```python
from build123d import *

# Parameters (mm, degrees)
SKETCH_1_W      = 27.5
SKETCH_1_H      = 13.5
EXTRUDE_1_DEPTH = 2.5
SKETCH_2_W      = 2.5
SKETCH_2_H      = 13.5
EXTRUDE_2_DEPTH = 3
SKETCH_3_R      = 0.25
EXTRUDE_3_DEPTH = 3
SKETCH_4_R      = 0.25
SKETCH_4_R_2    = 2.5
EXTRUDE_5_DEPTH = 20


with BuildPart() as part:
    # Эскиз1 → Бобышка-Вытянуть1 (new body)
    with BuildSketch(Plane(origin=(0, 0, 0), x_dir=(1, 0, 0), z_dir=(0, 1, 0))):
        Rectangle(SKETCH_1_W, SKETCH_1_H)
    extrude(amount=EXTRUDE_1_DEPTH)

    # Эскиз2 → Бобышка-Вытянуть2 (add)
    with BuildSketch(Plane.XZ):
        with Locations((12.5, 0)):
            Rectangle(SKETCH_2_W, SKETCH_2_H)
    extrude(amount=-EXTRUDE_2_DEPTH)

    # Эскиз3 → Бобышка-Вытянуть3 (add)
    with BuildSketch(Plane.ZY.offset(13.75)):
        with Locations(Location((1.75, 1.25, 0), (0, 0, 180))):
            Circle(SKETCH_3_R)
    extrude(amount=EXTRUDE_3_DEPTH)

    # Эскиз4 → Бобышка-Вытянуть5 (add)
    with BuildSketch(Plane.ZY.offset(16.75)):
        with Locations(Location((1.75, 1.25, 0), (0, 0, 180))):
            Circle(SKETCH_4_R)
        with Locations((-0.5, 1.25)):
            Circle(SKETCH_4_R_2)
        with Locations(Location((1.75, 1.25, 0), (0, 0, 180))):
            Circle(SKETCH_4_R)
    extrude(amount=EXTRUDE_5_DEPTH)


solid = part.part
```
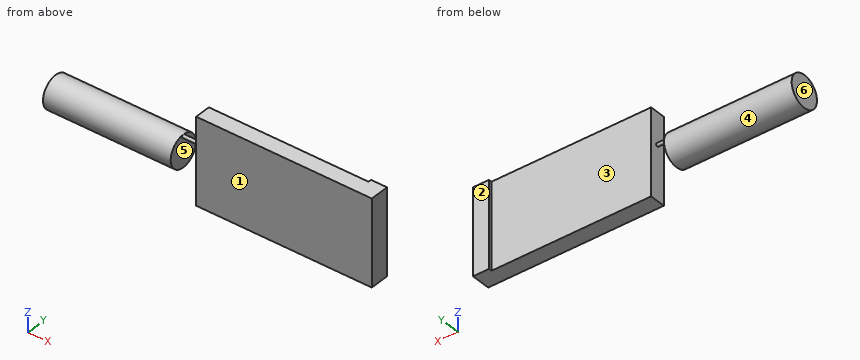
Geometry check sheet. Reference: the model listing, model coordinates, mm. Face numbers are marked on the shaded views. A direction names the side the tool comes from. Coordinates: 2 decimals unless noted, no trailing zeros. Order: outer loops, then holes, each group sorted by start corner. A loop starts at its lowest first (then second) coordinate and runs counter-clockwise, first axis right, second up.
Item 1: Scan lines: line 1 along Y through (x, z) = (-7.5, -3); line 2 along X through (y, z) = (1.8, 0.75); line 3 along X through (y, z) = (1.55, -5.5). Record each from-to range of solid material in increasing order.
Item 2: Depth check by flat-ended pin: pin 1 (2 mm diameter, centred on x = -25.5, y = 1.5, fed in from -Z); pin 2 (2 mm diameter, centred on x = -30.5, y = 3, fed in from -Z); pin 3 (7 mm diameter, centred on x = -1, z = -1.5, fed in from -Y); pin 4 (3 mm diameter, centred on x = -23.5, z = 5, fed in from +Y). Enter the tip coordinate at first touch or a pass-through.
Item 3: Section check A-A (z = -0.5). Enter the section's corners in (x, y).
Item 4: Tool access check on the marked faces 1, 2 and 3. Record the directions out of +Z, -Z, +X, -X, +Y, -Y that give a thin tool (end or side, any length) a straight path to the whole face; none if there is none.
Item 5: Section check D-D (x = -24). Enter the section's corners in (y, z).
Item 6: Section check B-B (z = -2.5). Enter the section's corners in (x, y), plus the area to 3 significant figures.
Item 7: Mould release check, pull along X, two halves, no side actions. Record for the marked faces 4, 5 and 6: released by +X, released by -X, zero draft, split by the parting line, or undercut.
Item 8: Section check C-C (y = 2). Enter the section's corners in (x, z), plus the area to 3 significant figures.
Check sheet entries:
1. line 1: y = 0 to 2.5
1. line 2: x = -36.75 to -16.75, -13.75 to 13.75
1. line 3: x = -13.75 to 13.75
2. pin 1: stops at z = -3
2. pin 2: stops at z = -2.88
2. pin 3: stops at y = 0
2. pin 4: passes through
3. outline: (-36.75, -1.25) - (-16.75, -1.25) - (-16.75, 3.75) - (-36.75, 3.75) - close; (-13.75, 0) - (13.75, 0) - (13.75, 3) - (11.25, 3) - (11.25, 2.5) - (-13.75, 2.5) - close
4. face 1: +Z, -Z, +X, -Y
4. face 2: +Z, -Z, +X, +Y
4. face 3: +Z, -Z, +Y
5. outline: circle Ø5 at (1.25, -0.5)
6. outline: (-36.75, -0.25) - (-16.75, -0.25) - (-16.75, 2.75) - (-36.75, 2.75) - close; (-13.75, 0) - (13.75, 0) - (13.75, 3) - (11.25, 3) - (11.25, 2.5) - (-13.75, 2.5) - close
6. area: 130 mm2
7. face 4: zero draft
7. face 5: undercut
7. face 6: released by -X
8. outline: (-36.75, -2.88) - (-16.75, -2.88) - (-16.75, 1.88) - (-36.75, 1.88) - close; (-13.75, -6.75) - (13.75, -6.75) - (13.75, 6.75) - (-13.75, 6.75) - close
8. area: 467 mm2
